```python
from build123d import *

# Parameters (mm, degrees)
F1_DEPTH = 7
F2_W     = 16
F2_H     = 7
F3_DEPTH = 10
F4_R     = 5
F5_R     = 3.49999
F6_R     = 18
F7_DEPTH = 3


# Not quite as in the source:
# - a fillet or chamfer is up to 0.001 mm smaller than in the source, because OpenCascade refuses the exact size


with BuildPart() as f1:
    # F0 (on Top) → F1 (new body)
    with BuildSketch(Plane.XY):
        with BuildLine():
            ThreePointArc((11, -16.7032930885), (17.6068168617, -9.4868329805), (20, 0))
            ThreePointArc((20, 0), (17.6068168617, 9.4868329805), (11, 16.7032930885))
            Line((11, 16.7032930885), (11, 12))
            Line((11, 12), (-11, 12))
            Line((-11, 12), (-11, 16.7032930885))
            ThreePointArc((-11, 16.7032930885), (-20, 0), (-11, -16.7032930885))
            Line((-11, -16.7032930885), (-11, -11.7698283494))
            Line((-11, -11.7698283494), (11, -11.7698283494))
            Line((11, -11.7698283494), (11, -16.7032930885))
        make_face()
        with BuildLine():
            Line((11, 12), (11, 16.7032930885))
            ThreePointArc((11, 16.7032930885), (0, 20), (-11, 16.7032930885))
            Line((-11, 16.7032930885), (-11, 12))
            Line((-11, 12), (11, 12))
        make_face()
        with BuildLine():
            ThreePointArc((-11, 16.7032930885), (0, 20), (11, 16.7032930885))
            Line((11, 16.7032930885), (11, 28))
            Line((11, 28), (-11, 28))
            Line((-11, 28), (-11, 16.7032930885))
        make_face()
        with BuildLine():
            Line((11, -28.2301716506), (11, -16.7032930885))
            ThreePointArc((11, -16.7032930885), (0, -20), (-11, -16.7032930885))
            Line((-11, -16.7032930885), (-11, -28.2301716506))
            Line((-11, -28.2301716506), (11, -28.2301716506))
        make_face()
        with BuildLine():
            ThreePointArc((-11, -16.7032930885), (0, -20), (11, -16.7032930885))
            Line((11, -16.7032930885), (11, -11.7698283494))
            Line((11, -11.7698283494), (-11, -11.7698283494))
            Line((-11, -11.7698283494), (-11, -16.7032930885))
        make_face()
    extrude(amount=F1_DEPTH)

    # F2 (on face) → F3 (cut)
    with BuildSketch(Plane.XY.offset(7)):
        with Locations((0, 24.5)):
            Rectangle(F2_W, F2_H)
        with Locations((0, -24.7301716506)):
            Rectangle(F2_W, F2_H)
    extrude(amount=-F3_DEPTH, mode=Mode.SUBTRACT)

    # F4
    f4_edges = [f1.edges().sort_by_distance(p)[0] for p in [
        (-8, 21, 3.5),
        (8, 21, 3.5),
        (8, -21.230172, 3.5),
        (-8, -21.230172, 3.5),
    ]]
    fillet(f4_edges, radius=F4_R)

    # F5 (radius 3.5 in the source; OpenCascade refuses exactly that, so slightly less here)
    f5_edges = [f1.edges().sort_by_distance(p)[0] for p in [
        (-9.5, -28.230172, 7),
        (9.5, -28.230172, 7),
        (-9.5, 28, 7),
        (9.5, 28, 7),
        (-9.5, 28, 0),
        (9.5, 28, 0),
        (-9.5, -28.230172, 0),
        (9.5, -28.230172, 0),
    ]]
    fillet(f5_edges, radius=F5_R)

    # F6 (on face) → F7 (join)
    with BuildSketch(Plane.XY.offset(7)):
        with BuildLine():
            Line((11, 16.7032930885), (11, 16.71100699))
            ThreePointArc((11, 16.71100699), (0, 20.0064428277), (-11, 16.71100699))
            Line((-11, 16.71100699), (-11, 16.7032930885))
            ThreePointArc((-11, 16.7032930885), (-20, 0), (-11, -16.7032930885))
            Line((-11, -16.7032930885), (-11, -16.71100699))
            ThreePointArc((-11, -16.71100699), (0, -20.0064428277), (11, -16.71100699))
            Line((11, -16.71100699), (11, -16.7032930885))
            ThreePointArc((11, -16.7032930885), (20, 0), (11, 16.7032930885))
        make_face()
        Circle(F6_R, mode=Mode.SUBTRACT)
    extrude(amount=F7_DEPTH)


solid = f1.part
```
Verification items for the finished model (mm, model axes). A direction names the side the tool comes from. Round coordinates to 2 decimals unless told otherwise and drop trailing zeros. Write each loop counter-clockwise with the first axis right and the second up, starting at its lowest first coordinate (ties: lowest second). Pieces come first, ordered by that corner, then holes. Notation, with made-up numbers: (-1.75, -32.5) -> (26.25, -32.5) arc R19 ccw to (26.25, -5.5) -> close; hole circle Ø11 at (-23, 30.25). An arc over 180 degrees is marked (long way). Write each question's results on one line, items separated by ' | '. Start each with the question number.
1. Set-up check for faces 4 (the flat face through (0, -21, 7)), 5 (the flat face through (-8, -27, 4)), 6 (the flat face through (-8, 27, 4)), 7 (the cylindrical face through (0.163, 20.006, 8.479)), 8 (the flat face through (11, -23, 4)): record each of +Z, -Z, +X, -X, +Y, -Y from which the full face is reachable in a straight line by a thin tool's end or side.
2. Depth check by flat-ended pin: P1, Ø2.5, axis at x = -5, y = -21.5, coming from the +Z side; P2, Ø0.6, axis at y = 26.5, z = 4.5, coming from the +X side; P3, Ø3, axis at x = -1, z = 4.5, coming from the -Y side. Enter the tip coordinate at first touch or a pass-through.
3. Cross-section at D-D (z = 5). Enter the section's corners in (x, y), then the cut area to 3 significant figures.
4. Material ranges on probe 1 along Y at (x, z) = (0, 7.85); probe 2 along Z at (x, y) = (10, -6); probe 3 along Y at (x, z) = (-2.5, 0.5), recorded low to high. Write a range as from..to.
5. Cross-section at B-B (x = 0). Enter the section's corners in (y, z), then the cut area to 3 significant figures.
6. Draft check along Y on faces 1 (the cylindrical face through (-0.163, -20.006, 8.479)), 2 (the flat face through (-11, -22, 3)), 3 (the flat face through (0, 0, 7)). Enter one of: +Y half, -Y half, draft (parallel to the pull), parting line (faces both ways), or undercut.
7. Cross-section at C-C (y = 3). Enter the section's corners in (x, z), then the cut area to 3 significant figures.
Solutions:
1) face 4: +Z, -Y | face 5: +Z, -Z, -Y | face 6: +Z, -Z, +Y | face 7: +Z, +Y | face 8: +Z, -Z, +X, -Y
2) P1: stops at z = 7 | P2: stops at x = 11 | P3: stops at y = -21.23
3) outline: (-11, -27.89) -> (-8, -27.89) -> (-8, -26.23) arc R5 cw to (-3, -21.23) -> (3, -21.23) arc R5 cw to (8, -26.23) -> (8, -27.89) -> (11, -27.89) -> (11, -16.7) arc R20 ccw to (11, 16.7) -> (11, 27.66) -> (8, 27.66) -> (8, 26) arc R5 cw to (3, 21) -> (-3, 21) arc R5 cw to (-8, 26) -> (-8, 27.66) -> (-11, 27.66) -> (-11, 16.7) arc R20 ccw to (-11, -16.7) -> close | area: 1,450 mm2
4) probe 1: y = -20.01..-18, 18..20.01 | probe 2: z = 0..7 | probe 3: y = -21.23..21
5) outline: (-21.23, 0) -> (21, 0) -> (21, 7) -> (20.01, 7) -> (20.01, 10) -> (18, 10) -> (18, 7) -> (-18, 7) -> (-18, 10) -> (-20.01, 10) -> (-20.01, 7) -> (-21.23, 7) -> close | area: 308 mm2
6) face 1: -Y half | face 2: draft | face 3: undercut
7) outline: (-19.77, 0) -> (19.77, 0) -> (19.77, 10) -> (17.75, 10) -> (17.75, 7) -> (-17.75, 7) -> (-17.75, 10) -> (-19.77, 10) -> close | area: 289 mm2
